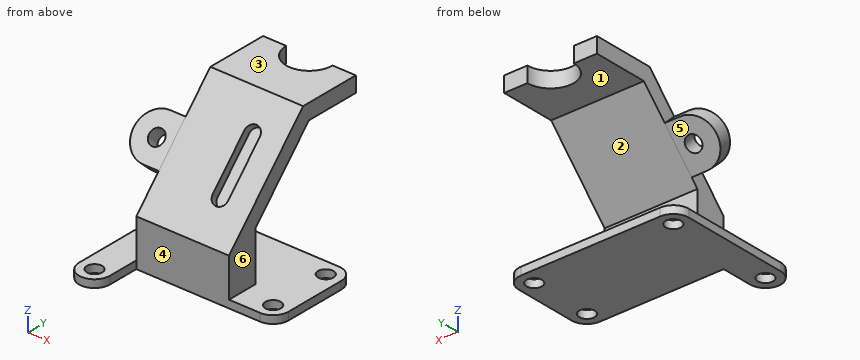
from build123d import *

# Parameters (mm, degrees)
F1_DEPTH  = 2
F3_DEPTH  = 24
F4_R      = 2
F5_DEPTH  = 2.001
F6_R      = 2
F7_DEPTH  = 4
F8_DEPTH  = 2
F10_DEPTH = 36.135672


with BuildPart() as f1:
    # F0 (on Top) → F1 (new body)
    with BuildSketch(Plane.XY):
        with BuildLine():
            Line((0, 28), (0, 0))
            ThreePointArc((0, 0), (4, -4), (8, 0))
            Line((8, 0), (8, 8))
            Line((8, 8), (40, 8))
            ThreePointArc((40, 8), (42.828427, 9.171573), (44, 12))
            Line((44, 12), (44, 28))
            ThreePointArc((44, 28), (42.828427, 30.828427), (40, 32))
            Line((40, 32), (4, 32))
            ThreePointArc((4, 32), (1.171573, 30.828427), (0, 28))
        make_face()
    extrude(amount=-F1_DEPTH)

    # F2 (on face) → F3 (join)
    with BuildSketch(Plane.YZ.offset(8)):
        Polygon((8, 10), (8, 0), (16, 0), (16, 12.713833), (32.245195, 30.134672), (46.505946, 30.134672), (46.505946, 34.134672), (30.505946, 34.134672), align=None)
    extrude(amount=F3_DEPTH)

    # F4 (on face) → F5 (cut, through all)
    with BuildSketch(Plane.XY):
        with Locations((40, 12)):
            Circle(F4_R)
        with Locations((40, 28)):
            Circle(F4_R)
        with Locations((4, 0)):
            Circle(F4_R)
        with Locations((4, 28)):
            Circle(F4_R)
    extrude(amount=-F5_DEPTH, mode=Mode.SUBTRACT)

    # F6 (on face) → F7 (join)
    with BuildSketch(Plane(origin=(0, -0.708794, 0.660961), x_dir=(1, 0, 0), z_dir=(0, -0.731354, 0.681998))):
        with BuildLine():
            Line((4, 22.769524), (8, 22.769524))
            Line((8, 22.769524), (8, 34.769524))
            Line((8, 34.769524), (4, 34.769524))
            ThreePointArc((4, 34.769524), (-2, 28.769524), (4, 22.769524))
        make_face()
        with Locations((4, 28.769524)):
            Circle(F6_R, mode=Mode.SUBTRACT)
    extrude(amount=-F7_DEPTH)

    # F6 (on face) → F8 (cut)
    with BuildSketch(Plane(origin=(0, -0.708794, 0.660961), x_dir=(1, 0, 0), z_dir=(0, -0.731354, 0.681998))):
        with BuildLine():
            Line((26, 22.769524), (26, 36.769524))
            ThreePointArc((26, 36.769524), (24, 38.769524), (22, 36.769524))
            Line((22, 36.769524), (22, 22.769524))
            ThreePointArc((22, 22.769524), (24, 20.769524), (26, 22.769524))
        make_face()
    extrude(amount=-F8_DEPTH, mode=Mode.SUBTRACT)

    # F9 (on face) → F10 (cut, through all)
    with BuildSketch(Plane.XY.offset(34.134672)):
        with BuildLine():
            ThreePointArc((14, 46.505946), (20, 40.505946), (26, 46.505946))
            Line((26, 46.505946), (14, 46.505946))
        make_face()
    extrude(amount=-F10_DEPTH, mode=Mode.SUBTRACT)


solid = f1.part
CAD build for the part. Positions are in the model's coordinates, mm. Face numbers are marked on the shaded views. A direction names the side the tool comes from. Give positions to 0.01 mm unless a question says otherwise; leave off trailing zeros. Order: outer loops, then holes, each group sorted by start corner. A loop starts at its lowest first (then second) coordinate and runs counter-clockwise, first axis right, second up. Notation, with made-up numbers: (72, -25) - (105, -25) arc R19 cw to (105, -17) - close; hole circle Ø3 at (68.5, 80). An arc over 180 degrees is marked (long way). Answer in a Markdown table with one row per item.
1. Pull direction Z, two halves, no side cores. Call the marked faces 1, 2 and 3: pulls with the +Z half, pulls with the -Z half, needs draft (parallel to the pull), parting line crosses it, or undercut.
Data:
| item | result |
|---|---|
| face 1 | pulls with the -Z half |
| face 2 | undercut |
| face 3 | pulls with the +Z half |
2. Probe probe 1 along Y at (x, z) = (4, -1.3); probe 2 along Y at (x, z) = (40, -1); probe 3 along Z at (x, y) = (16, 29). List the from-to ranges inside material, lowest first. Write a range as [from, to].
Data:
| item | result |
|---|---|
| probe 1 | y = [-4, -2], [2, 26], [30, 32] |
| probe 2 | y = [8, 10], [14, 26], [30, 32] |
| probe 3 | z = [-2, 0], [26.65, 32.52] |
3. Saw through at B-B, the plane z = 5.5. Give the cut face in (x, y), plus the area to 3 significant figures.
Data:
| item | result |
|---|---|
| outline | (8, 8) - (32, 8) - (32, 16) - (8, 16) - close |
| area | 192 mm² |
4. Saw through at A-A, the plane x = 9.5. Give the cut face in (y, z).
Data:
| item | result |
|---|---|
| outline | (8, -2) - (32, -2) - (32, 0) - (16, 0) - (16, 12.71) - (32.25, 30.13) - (46.51, 30.13) - (46.51, 34.13) - (30.51, 34.13) - (8, 10) - close |
5. Saw through at D-D, the plane x = 20. Give the cut face in (y, z).
Data:
| item | result |
|---|---|
| outline | (8, -2) - (32, -2) - (32, 0) - (16, 0) - (16, 12.71) - (32.25, 30.13) - (40.51, 30.13) - (40.51, 34.13) - (30.51, 34.13) - (8, 10) - close |
6. Flat gauge pins, fed straight in: pin 1 (1 mm diameter, centred on x = 31, y = 10.5, fed in from +Z); pin 2 (1 mm diameter, centred on x = 14.5, z = -1, fed in from +Y); pin 3 (3.5 mm diameter, centred on x = 20.5, z = 4.5, fed in from -Y). Where does each tip first touch, or does it go through?
Data:
| item | result |
|---|---|
| pin 1 | stops at z = 13.22 |
| pin 2 | stops at y = 32 |
| pin 3 | stops at y = 8 |
7. Saw through at C-C, the plane y = 9. Give the cut face in (x, z), plus the area to 3 significant figures.
Data:
| item | result |
|---|---|
| outline | (0, -2) - (42.65, -2) - (42.65, 0) - (32, 0) - (32, 11.07) - (8, 11.07) - (8, 0) - (0, 0) - close |
| area | 351 mm² |
8. Tool access for the marked faces 4, 5 and 6: list every direction of +Z, -Z, +X, -X, +Y, -Y with a clear straight run to the whole face (end or side of a thin tool).
Data:
| item | result |
|---|---|
| face 4 | +Z, -Z, +X, -Y |
| face 5 | +X, -X, +Y |
| face 6 | +Z, +X, +Y, -Y |
